Check sheet for the modelled part. Datum: model origin and axes. Units: mm. A direction names the side the tool comes from. Round coordinates to 2 decimals unless told otherwise and drop trailing zeros. Write each loop counter-clockwise with the first axis right and the second up, starting at its lowest first coordinate (ties: lowest second). Pieces come first, ordered by that corner, then holes.
from build123d import *

# Parameters (mm, degrees)
SKETCH1_R               = 4.7625
BOSS_EXTRUDE1_DEPTH     = 9.525
SKETCH2_R               = 38.1
BOSS_EXTRUDE2_DEPTH     = 2.54
CUT_EXTRUDE1_DEPTH      = 55.716959208
CUT_EXTRUDE1_DEPTH_BACK = 55.716959208


with BuildPart() as part:
    # Sketch1 → Boss-Extrude1 (new body)
    with BuildSketch(Plane(origin=(0, 0, 0), x_dir=(0, 0, -1), z_dir=(1, 0, 0))):
        with Locations(Location((0, 0, 0), (0, 0, 180))):
            Circle(SKETCH1_R)
        with BuildLine():
            Line((-1.905, -1.956171069), (-1.905, 1.956171069))
            ThreePointArc((-1.905, 1.956171069), (0, 2.7305), (1.905, 1.956171069))
            Line((1.905, 1.956171069), (1.905, -1.956171069))
            ThreePointArc((1.905, -1.956171069), (0, -2.7305), (-1.905, -1.956171069))
        make_face(mode=Mode.SUBTRACT)
    extrude(amount=BOSS_EXTRUDE1_DEPTH)

    # Sketch2 → Boss-Extrude2 (add)
    with BuildSketch(Plane.ZY):
        Circle(SKETCH2_R)
    extrude(amount=BOSS_EXTRUDE2_DEPTH)

    # Sketch3 → Cut-Extrude1 (cut, two sides: drawn at the far end of the back side and taken through both)
    with BuildSketch(Plane(origin=(0, 0, 0), x_dir=(0, 0, -1), z_dir=(1, 0, 0)).offset(-CUT_EXTRUDE1_DEPTH_BACK)):
        Polygon((-3.175, 10.261761314), (0, 4.7625), (3.175, 10.261761314), (3.175, 38.1), (-3.175, 38.1), align=None)
    extrude(amount=CUT_EXTRUDE1_DEPTH + CUT_EXTRUDE1_DEPTH_BACK, mode=Mode.SUBTRACT)


solid = part.part
1. Sectioned sample at A-A, the plane y = 9. Enter the section's corners in (x, z).
2. Scan lines: line 1 along X through (y, z) = (4.5, 8); line 2 along Z through (x, y) = (-1.25, 33.5) (3 decimals); line 3 along Y through (x, z) = (-0.75, -20). Record each from-to range of solid material in increasing order.
3. Go/stop test with flat-tipped pins: pin 1 (5 mm diameter, centred on x = 4, z = 1.5, fed in from +Y); pin 2 (1.2 mm diameter, centred on x = 3, y = 1, fed in from -Z); pin 3 (2 mm diameter, centred on x = -1, y = 29, fed in from -Z). Record where each tip stops, or that it passes through.
4. Sectioned sample at C-C, the plane y = 0. Enter the section's corners in (x, z) (1 decimal), plus the area to 3 significant figures.
5. Sectioned sample at D-D, the plane z = 6. Enter the section's corners in (x, y), plus the area to 3 significant figures.
6. Sectioned sample at B-B, the plane x = 3. Enter the section's corners in (y, z) (1 decimal).
7. Release check for a two-part mould opening along Y. For faces 1 (the cylindrical face through (4.7, 4.65, -1.03)), 2 (the flat face through (-1.29, 7.55, 1.61)), 3 (the flat face through (-1, 24, -3.175)), 4 (the flat face through (5, 0, -1.905)) record: released by +Y, released by -Y, zero draft, split by the parting line, or undercut.
8. Set-up check for faces 5 (the flat face through (-1.288, 7.474, -1.565)), 6 (the cylindrical face through (4.7, -2.73, -0.03)), 7 (the flat face through (-2.54, 0, -1)): record each of +Z, -Z, +X, -X, +Y, -Y from which the full face is reachable in a straight line by a thin tool's end or side.
Computed values:
1. outline: (-2.54, -37.02) - (0, -37.02) - (0, -2.45) - (-2.54, -2.45) - close; (-2.54, 2.45) - (0, 2.45) - (0, 37.02) - (-2.54, 37.02) - close
2. line 1: x = -2.54 to 0
2. line 2: z = -18.148 to -3.175, 3.175 to 18.148
2. line 3: y = -32.43 to 32.43
3. pin 1: stops at y = 4.76
3. pin 2: stops at z = -4.75
3. pin 3: stops at z = -25.84
4. outline: (-2.5, -38.1) - (0, -38.1) - (0, -4.8) - (9.5, -4.8) - (9.5, -1.9) - (0, -1.9) - (0, 1.9) - (9.5, 1.9) - (9.5, 4.8) - (0, 4.8) - (0, 38.1) - (-2.5, 38.1) - close
4. area: 248 mm2
5. outline: (-2.54, -37.62) - (0, -37.62) - (0, 37.62) - (-2.54, 37.62) - close
5. area: 191 mm2
6. outline: circle Ø9.5 at (0, 0); hole (-2, -1.9) - (2, -1.9) arc R2.7 ccw to (2, 1.9) - (-2, 1.9) arc R2.7 ccw to start
7. face 1: split by the parting line
7. face 2: released by +Y
7. face 3: zero draft
7. face 4: undercut
8. face 5: +X, -X, +Y
8. face 6: +X
8. face 7: +Z, -Z, -X, +Y, -Y
